Part print with two shaded views. Sizes in mm from the minimum x, y, z corner. Coordinates: 2 decimals unless noted, no trailing zeros. Order: outer loops, then holes, each group sorted by start corner. A loop starts at its lowest first (then second) coordinate and runs counter-clockwise, first axis right, second up.
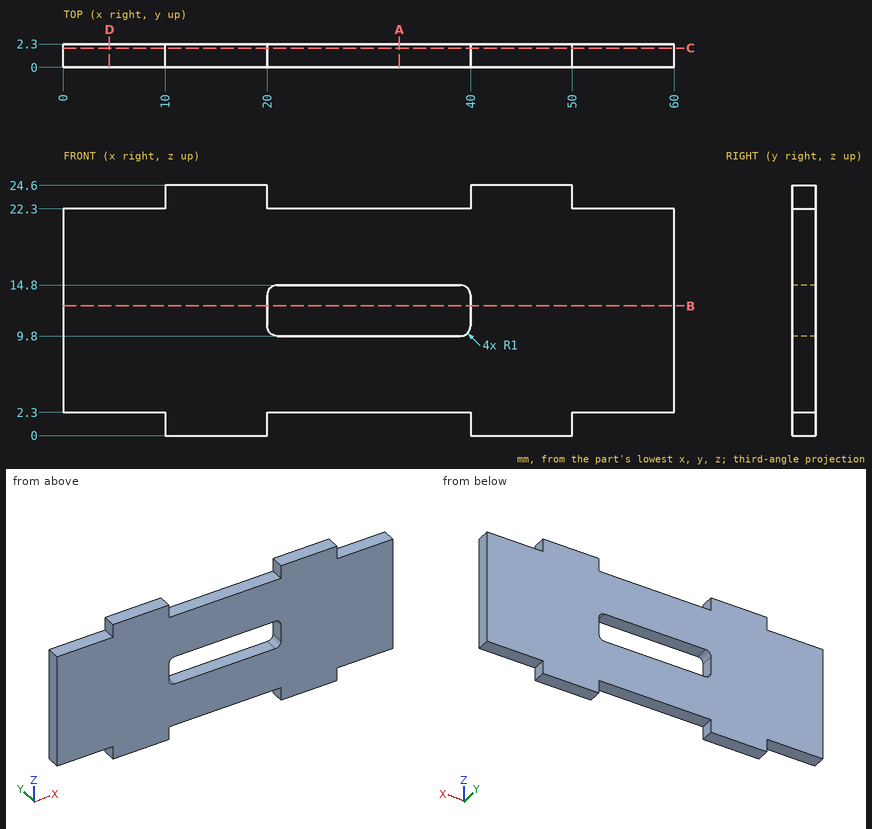
Q1. Cut at C-C on y = 1.9. Write the cut outline in (x, z).
Results list:
outline: (0, 2.3) - (10, 2.3) - (10, 0) - (20, 0) - (20, 2.3) - (40, 2.3) - (40, 0) - (50, 0) - (50, 2.3) - (60, 2.3) - (60, 22.3) - (50, 22.3) - (50, 24.6) - (40, 24.6) - (40, 22.3) - (20, 22.3) - (20, 24.6) - (10, 24.6) - (10, 22.3) - (0, 22.3) - close; hole (20, 10.8) arc R1 ccw to (21, 9.8) - (39, 9.8) arc R1 ccw to (40, 10.8) - (40, 13.8) arc R1 ccw to (39, 14.8) - (21, 14.8) arc R1 ccw to (20, 13.8) - close
Q2. Cut at A-A on x = 33. Write the cut outline in (y, z), and give its area (3 significant figures).
Results list:
outline: (0, 2.3) - (2.3, 2.3) - (2.3, 9.8) - (0, 9.8) - close; (0, 14.8) - (2.3, 14.8) - (2.3, 22.3) - (0, 22.3) - close
area: 34.5 mm2
Q3. Cut at D-D on x = 4.5. Write the cut outline in (y, z).
Results list:
outline: (0, 2.3) - (2.3, 2.3) - (2.3, 22.3) - (0, 22.3) - close
Q4. Pin check, flat tips, straight feed: pin 1 Ø1.2 at (y, z) = (1.5, 0.5) entering from +X; pin 2 Ø1.2 at (y, z) = (1, 24) entering from -X; pin 3 Ø0.7 at (x, y) = (56.5, 1) entering from +Z. Stop position of each tip, or through.
Results list:
pin 1: stops at x = 50
pin 2: stops at x = 10
pin 3: stops at z = 22.3
Q5. Cut at B-B on z = 12.75. Write the cut outline in (x, y), and give its area (3 significant figures).
Results list:
outline: (0, 0) - (20, 0) - (20, 2.3) - (0, 2.3) - close; (40, 0) - (60, 0) - (60, 2.3) - (40, 2.3) - close
area: 92.0 mm2
Q6. Wall check: line 1 along X through (y, z) = (1, 23.5); line 2 along Z through (x, y) = (29, 0.4); line 3 along X through (y, z) = (2.25, 13.25). Give the ranges that are in metal, low to high.
Results list:
line 1: x = 10 to 20, 40 to 50
line 2: z = 2.3 to 9.8, 14.8 to 22.3
line 3: x = 0 to 20, 40 to 60
